```python
from build123d import *

# Parameters (mm, degrees)
F0_W            = 100
F0_H            = 100
F2_DEPTH        = 25
F4_DEPTH        = 25.001
F4_COPIES_COUNT = 4


# Not quite as in the source:
# - a pattern or mirror of a feature is missing from the dataset's text; its kind, count and spacing are read off the source's solid


with BuildPart() as f2:
    # F0 (on Front) → F2 (new body)
    with BuildSketch(Plane.XZ):
        Rectangle(F0_W, F0_H)
    extrude(amount=F2_DEPTH)

    # F3 (on Front) → F4 (cut, through all)
    with BuildSketch(Plane.XZ):
        Polygon((7.5, 50), (0, 50), (-7.5, 50), (-7.5, 45), (-12.5, 45), (-12.5, 40), (0, 40), (12.5, 40), (12.5, 45), (7.5, 45), align=None)
    f4 = extrude(amount=F4_DEPTH, mode=Mode.SUBTRACT)

    # F4_copies: F4 ×4 about axis
    f4_copies_axis = Axis((0, 0, 0), (0, 1, 0))
    for i in range(1, F4_COPIES_COUNT):
        add(f4.rotate(f4_copies_axis, i * 360 / F4_COPIES_COUNT), mode=Mode.SUBTRACT)


solid = f2.part
```
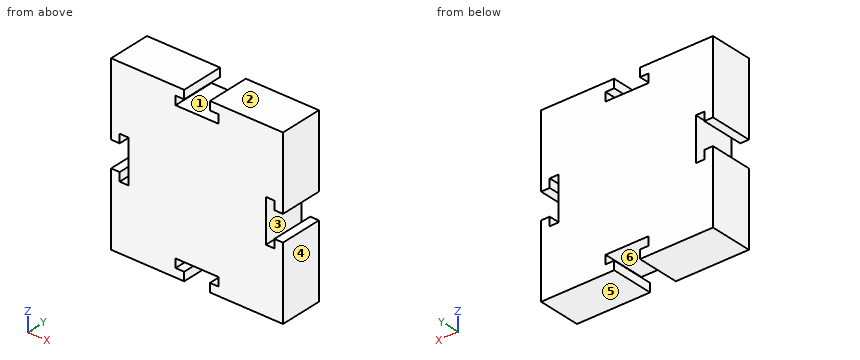
Design review of the part built by this model. Coordinates are the model's own, in mm. Face numbers are marked on the shaded views. A direction names the side the tool comes from. Round coordinates to 2 decimals unless told otherwise and drop trailing zeros. Write each loop counter-clockwise with the first axis right and the second up, starting at its lowest first coordinate (ties: lowest second). Pieces come first, ordered by that corner, then holes. Notation, with made-up numbers: (32, 87.25) -> (83, 87.25) arc R33 ccw to (83, 119.25) -> close; hole circle Ø7 at (83.5, 5). An arc over 180 degrees is marked (long way). Answer in a Markdown table with one row per item.
Q1. To check wall thickness, follow L1, parallel to X at y = -11.75, z = -8.5; L2, parallel to X at y = -7, z = 43.5. State the ranges of each line that lie inside material, in increasing order. Write a range as [from, to].
The answers:
| item | result |
|---|---|
| L1 | [-50, -45], [-40, 40], [45, 50] |
| L2 | [-50, -12.5], [12.5, 50] |
Q2. Take a section at A-A, the plane z = 43.5. State the section outline as (x, y) points.
The answers:
| item | result |
|---|---|
| outline | (-50, -25) -> (-12.5, -25) -> (-12.5, 0) -> (-50, 0) -> close; (12.5, -25) -> (50, -25) -> (50, 0) -> (12.5, 0) -> close |
Q3. For the marked faces 5 and 6, list the 3-axis set-ups (+Z, -Z, +X, -X, +Y, -Y) from which the entire face can be reached by the end or side of a thin tool; tool diameter is ignored.
The answers:
| item | result |
|---|---|
| face 5 | -Z, +X, -X, +Y, -Y |
| face 6 | +Y, -Y |
Q4. Clearance check with flat-ended pins moving along their axes: pin 1 Ø1.5 at (x, y) = (6, -7) entering from -Z; pin 2 Ø8 at (x, z) = (-24, 19) entering from +Y. State where each tip first meets the part, or that it passes through.
The answers:
| item | result |
|---|---|
| pin 1 | z = -40 |
| pin 2 | y = 0 |
Q5. Draft analysis for pull direction Z (two halves, no side actions). For the marked faces 1, 2, 3 and 4, state which applies: +Z half, -Z half, draft (parallel to the pull), parting line (faces both ways), or undercut.
The answers:
| item | result |
|---|---|
| face 1 | undercut |
| face 2 | +Z half |
| face 3 | undercut |
| face 4 | draft |
Q6. Take a section at C-C, the plane x = 4.5. State the section outline as (y, z) points, then the cut area to 3 significant figures.
The answers:
| item | result |
|---|---|
| outline | (-25, -40) -> (0, -40) -> (0, 40) -> (-25, 40) -> close |
| area | 2,000 mm² |
Q7. Take a section at B-B, the plane z = -10.5. State the section outline as (x, y) points.
The answers:
| item | result |
|---|---|
| outline | (-50, -25) -> (-45, -25) -> (-45, 0) -> (-50, 0) -> close; (-40, -25) -> (40, -25) -> (40, 0) -> (-40, 0) -> close; (45, -25) -> (50, -25) -> (50, 0) -> (45, 0) -> close |
